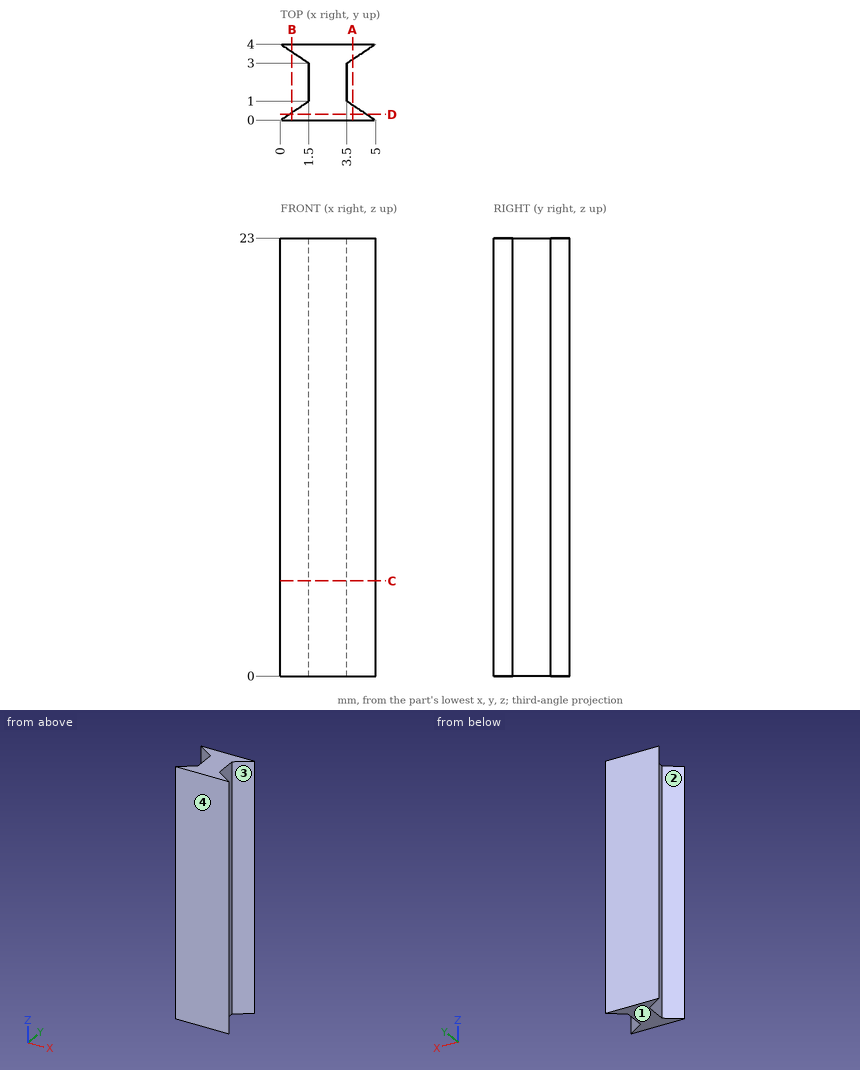
The figure shows three views and two pictorial views of one solid part (mm, origin at its lowest corner). Answer the questions. Round coordinates to 2 decimals unless told otherwise and drop trailing zeros. Write each loop counter-clockwise with the first axis right and the second up, starting at its lowest first coordinate (ties: lowest second). Pieces come first, ordered by that corner, then holes. Notation, with made-up numbers: (-12.5, -39.5) -> (-5.5, -39.5) arc R24 ccw to (-5.5, -27.5) -> close; hole circle Ø6 at (-26.75, 14). An arc over 180 degrees is marked (long way). Answer as a JSON object with one key per item and string values. Group by question number.
Q1. Section C-C (z = 5) is taken. Write down the section's boundary in (x, y).
Q2. Determine the mould class of the marked faces 1, 2, 3 and 4 for opening direction Y: pulls with the +Y half, pulls with the -Y half, needs draft (parallel to the pull), parting line crosses it, or undercut.
Q3. Section A-A (x = 3.8) is taken. Write down the section's boundary in (y, z).
Q4. Section B-B (x = 0.6) is taken. Write down the section's boundary in (y, z).
Q5. Section D-D (y = 0.3) is taken. Write down the section's boundary in (x, z).
Q6. This flat-tipped pin is pushed along its axis until it touches: pin 1 Ø2 at (y, z) = (2.5, 12) entering from -X. Where does it stop, or does it pass through?
Q7. Straight lines are drawn through the part: line 1 along X through (y, z) = (1.7, 5.25); line 2 along Y through (x, z) = (0.9, 2); line 3 along Y through (x, z) = (1.4, 3.5). For each, find the intervals that lie inside material, in ascending order.
Check values:
{
 "1": {"outline": "(0, 0) -> (5, 0) -> (3.5, 1) -> (3.5, 3) -> (5, 4) -> (0, 4) -> (1.5, 3) -> (1.5, 1) -> close"},
 "2": {"face 1": "needs draft", "face 2": "undercut", "face 3": "undercut", "face 4": "pulls with the -Y half"},
 "3": {"outline": "(0, 0) -> (0.8, 0) -> (0.8, 23) -> (0, 23) -> close; (3.2, 0) -> (4, 0) -> (4, 23) -> (3.2, 23) -> close"},
 "4": {"outline": "(0, 0) -> (0.4, 0) -> (0.4, 23) -> (0, 23) -> close; (3.6, 0) -> (4, 0) -> (4, 23) -> (3.6, 23) -> close"},
 "5": {"outline": "(0.45, 0) -> (4.55, 0) -> (4.55, 23) -> (0.45, 23) -> close"},
 "6": {"pin 1": "x = 0.75"},
 "7": {"line 1": "1.5 to 3.5", "line 2": "0 to 0.6, 3.4 to 4", "line 3": "0 to 0.93, 3.07 to 4"}
}
